Verification items for the finished model (mm, model axes). Face numbers are marked on the shaded views. A direction names the side the tool comes from. Coordinates: 2 decimals unless noted, no trailing zeros. Order: outer loops, then holes, each group sorted by start corner. A loop starts at its lowest first (then second) coordinate and runs counter-clockwise, first axis right, second up. Notation, with made-up numbers: M 54.25,39.25 L 77.25,39.25 A20 ccw 77.25,50.25 Z; hole C 51,-20 d2. An arc over 180 degrees is marked long. Return JSON: item names as keys, results as strings. Group by question number.
Q1. Go/stop test with flat-tipped pins: pin 1 Ø5.5 at (y, z) = (98.5, -8) entering from +X; pin 2 Ø1.5 at (y, z) = (97.5, 8) entering from -X; pin 3 Ø3 at (y, z) = (-16, -4) entering from -X; pin 4 Ø14.5 at (x, y) = (0, 10) entering from +Z. Record where each tip stops, or that it passes through.
Q2. Access from +Z, -Z, +X, -X, +Y, -Y to the whole of each face (thin tool, end or side, straight path). Record for the marked faces 4 and 5.
Q3. Section check C-C, the plane z = 7.75. Enter the section's corners in (x, y), then the cut area to 3 significant figures.
Q4. Section check D-D, the plane y = 103.5. Enter the section's corners in (x, z), then the cut area to 3 significant figures.
Q5. Thickness scan on probe 1 along Y at (x, z) = (0, -2.25); probe 2 along X at (y, z) = (103, 7); probe 3 along Y at (x, z) = (-2.5, 3). Record the ranges inside material, lowest first.
Q6. Mould release check, pull along Y, two halves, no side actions. Record for the marked faces 1, 2 and 3: pulls with the +Y half, pulls with the -Y half, needs draft (parallel to the pull), parting line crosses it, or undercut.
Q7. Section check B-B, the plane z = -2.5. Enter the section's corners in (x, y), then the cut area to 3 significant figures.
Q8. Section check A-A, the plane x = 0. Enter the section's corners in (y, z), then the cut area to 3 significant figures.
from build123d import *

# Parameters (mm, degrees)
BOSS_EXTRUDE1_DEPTH = 10
BOSS_EXTRUDE2_DEPTH = 5


with BuildPart() as part:
    # Sketch1 → Boss-Extrude1 (new, symmetric)
    with BuildSketch(Plane.XY):
        with BuildLine():
            Line((22, 110), (22, 82))
            ThreePointArc((22, 82), (0, 60), (-22, 82))
            Line((-22, 82), (-22, 110))
            ThreePointArc((-22, 110), (0, 132), (22, 110))
        make_face()
        with BuildLine():
            Line((10, 96), (10, 110))
            ThreePointArc((10, 110), (0, 120), (-10, 110))
            Line((-10, 110), (-10, 96))
            ThreePointArc((-10, 96), (-11.070466269, 95.802517077), (-12, 95.236067977))
            Line((-12, 95.236067977), (-12, 82))
            ThreePointArc((-12, 82), (0, 70), (12, 82))
            Line((12, 82), (12, 95.236067977))
            ThreePointArc((12, 95.236067977), (11.070466269, 95.802517077), (10, 96))
        make_face(mode=Mode.SUBTRACT)
    extrude(amount=BOSS_EXTRUDE1_DEPTH, both=True)

    # Sketch1_3 → Boss-Extrude2 (add, symmetric)
    with BuildSketch(Plane.XY):
        with BuildLine():
            Line((-20.54909502, 117.857142857), (-29.889592756, 93.428571429))
            ThreePointArc((-29.889592756, 93.428571429), (-31.795758241, 78.390324411), (-26.567056796, 64.162077105))
            ThreePointArc((-26.567056796, 64.162077105), (-21.561800954, 45.141212789), (-29.413527167, 27.108013937))
            ThreePointArc((-29.413527167, 27.108013937), (0, -40), (29.413527167, 27.108013937))
            ThreePointArc((29.413527167, 27.108013937), (21.561800954, 45.141212789), (26.567056796, 64.162077105))
            ThreePointArc((26.567056796, 64.162077105), (31.795758241, 78.390324411), (29.889592756, 93.428571429))
            Line((29.889592756, 93.428571429), (20.54909502, 117.857142857))
            ThreePointArc((20.54909502, 117.857142857), (21.634233178, 113.994991212), (22, 110))
            Line((22, 110), (22, 82))
            ThreePointArc((22, 82), (0, 60), (-22, 82))
            Line((-22, 82), (-22, 110))
            ThreePointArc((-22, 110), (-21.634233178, 113.994991212), (-20.54909502, 117.857142857))
        make_face()
        with BuildLine():
            ThreePointArc((-11.878172589, 8.294416244), (-11.969504398, 9.1450354), (-12, 10))
            ThreePointArc((-12, 10), (0, 22), (12, 10))
            ThreePointArc((12, 10), (11.969504398, 9.1450354), (11.878172589, 8.294416244))
            Line((11.878172589, 8.294416244), (10, -18))
            ThreePointArc((10, -18), (0, -28), (-10, -18))
            Line((-10, -18), (-11.878172589, 8.294416244))
        make_face(mode=Mode.SUBTRACT)
    extrude(amount=BOSS_EXTRUDE2_DEPTH, both=True)


solid = part.part
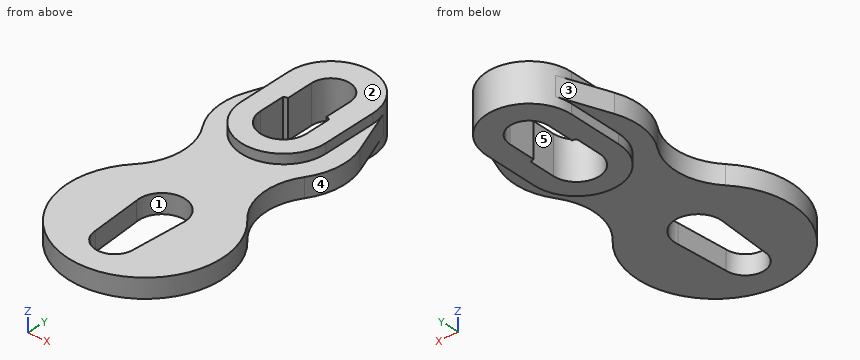
Numbers:
{
 "1": {"pin 1": "stops at x = 22", "pin 2": "stops at x = -22", "pin 3": "stops at x = -37.28", "pin 4": "passes through"},
 "2": {"face 4": "+Z, -Z, +X", "face 5": "+Z, -Z"},
 "3": {"outline": "M -22,82 A22 ccw 22,82 L 22,110 A22 ccw -22,110 Z; hole M -12,82 A12 ccw 12,82 L 12,95.24 A3 ccw 10,96 L 10,110 A10 ccw -10,110 L -10,96 A3 ccw -12,95.24 Z", "area": "1,750 mm2"},
 "4": {"outline": "M -26.04,-5 L -22,-5 L -22,-10 L -10,-10 L -10,10 L -22,10 L -22,5 L -26.04,5 Z; M 10,-10 L 22,-10 L 22,-5 L 26.04,-5 L 26.04,5 L 22,5 L 22,10 L 10,10 Z", "area": "561 mm2"},
 "5": {"probe 1": "y = -40 to -28, 22 to 70, 120 to 132", "probe 2": "x = -22 to -10, 10 to 22", "probe 3": "y = -39.92 to -27.68, 21.74 to 70.26, 119.68 to 131.86"},
 "6": {"face 1": "undercut", "face 2": "needs draft", "face 3": "pulls with the +Y half"},
 "7": {"outline": "M -29.89,93.43 A32 ccw -26.57,64.16 A30 cw -29.41,27.11 A40 ccw long 29.41,27.11 A30 cw 26.57,64.16 A32 ccw 29.89,93.43 L 20.55,117.86 A22 ccw -20.55,117.86 Z; hole M -12,82 A12 ccw 12,82 L 12,95.24 A3 ccw 10,96 L 10,110 A10 ccw -10,110 L -10,96 A3 ccw -12,95.24 Z; hole M -11.88,8.29 L -10,-18 A10 ccw 10,-18 L 11.88,8.29 A12 ccw long Z", "area": "7,700 mm2"},
 "8": {"outline": "M -40,-5 L -28,-5 L -28,5 L -40,5 Z; M 22,-5 L 60,-5 L 60,-10 L 70,-10 L 70,10 L 60,10 L 60,5 L 22,5 Z; M 120,-10 L 132,-10 L 132,10 L 120,10 Z", "area": "940 mm2"}
}
